```python
from build123d import *

# Parameters (mm, degrees)
EXTRUDE_DEPTH = 3.3
SKETCH001_R   = 1.5
POCKET_DEPTH  = 3.301
PAD_DEPTH     = 1


with BuildPart() as part:
    # Sketch → Extrude (new body)
    with BuildSketch(Plane.XY):
        with BuildLine():
            ThreePointArc((3.5, 21.5), (0, 25), (-3.5, 21.5))
            Line((-3.5, 21.5), (-3.5, 19.691369))
            ThreePointArc((-3.5, 19.691369), (0, -20), (3.5, 19.691369))
            Line((3.5, 19.691369), (3.5, 21.5))
        make_face()
    extrude(amount=EXTRUDE_DEPTH)

    # Sketch001 (on Face6 of Extrude) → Pocket (cut, through all)
    with BuildSketch(Plane.XY.offset(3.3)):
        with Locations((0, 21.5)):
            Circle(SKETCH001_R)
    extrude(amount=-POCKET_DEPTH, mode=Mode.SUBTRACT)

    # Sketch002 (on Face1 of CopyClone) → Pad (join)
    with BuildSketch(Plane.XY.offset(3.3)):
        with BuildLine():
            Line((-1.5, 13.5), (-1.5, -5))
            ThreePointArc((-1.5, -5), (0, -6.5), (1.5, -5))
            Line((1.5, 13.5), (1.5, -5))
            ThreePointArc((1.5, 13.5), (0, 14.581139), (-1.5, 13.5))
        make_face()
        with BuildLine():
            Line((-3.2, 9.765466), (-3.2, 6.765466))
            ThreePointArc((-3.2, 6.765466), (0, -10.943698), (3.2, 6.765466))
            Line((3.2, 9.765466), (3.2, 6.765466))
            ThreePointArc((-3.2, 9.765466), (0, -13.8), (3.2, 9.765466))
        make_face()
    extrude(amount=PAD_DEPTH)


solid = part.part
```
Build history of the part. All positions in model axes, mm. A direction names the side the tool comes from. Give positions to 0.01 mm unless a question says otherwise; leave off trailing zeros. Order: outer loops, then holes, each group sorted by start corner. A loop starts at its lowest first (then second) coordinate and runs counter-clockwise, first axis right, second up. Notation, with made-up numbers: M -39.75,55 L -12.75,55 A24 ccw -12.75,74 Z; hole C 70.5,76 d10. An arc over 180 degrees is marked long. Return JSON: item names as keys, results as strings.
Q1. 3-axis set-ups, long thin cutter, end or side, ignore diameter. For faces 4 (the face through (-0.83, -19.983, 1.627)), 5 (the face through (3.2, 8, 4)), 6 (the face through (-3.5, 21, 2)), 7 (the face through (-0.48, -13.79, 3.79)): which of +Z, -Z, +X, -X, +Y, -Y reach the whole face in a straight line?
Answer list:
{"face 4": "+Z, -Z", "face 5": "+Z, +Y", "face 6": "+Z, -Z, -X, +Y", "face 7": "+Z"}
Q2. Wall check: probe 1 along X at (y, z) = (-1.8, 3.75); probe 2 along Y at (x, z) = (0, 1.1); probe 3 along Z at (x, y) = (-6.5, 1). Give the ranges that are in metal, low to high. Write a range as from..to.
Answer list:
{"probe 1": "x = -12..-9.14, -1.5..1.5, 9.14..12", "probe 2": "y = -20..20, 23..25", "probe 3": "z = 0..3.3"}
Q3. Flat gauge pins, fed straight in: pin 1 (12 mm diameter, centred on x = 3.5, y = -13.5, fed in from -Z); pin 2 (0.5 mm diameter, centred on y = 20.5, z = 2, fed in from +X); pin 3 (0.5 mm diameter, centred on y = 8.5, z = 4, fed in from +X); pin 4 (0.5 mm diameter, centred on y = 6, z = 4, fed in from -X). Where does each tip first touch, or does it go through?
Answer list:
{"pin 1": "stops at z = 0", "pin 2": "stops at x = 3.5", "pin 3": "stops at x = 6.56", "pin 4": "stops at x = -9.33"}
Q4. Band-saw the part on D-D (x = -11). Give the cut face in (y, z).
Answer list:
{"outline": "M -16.7,0 L 16.7,0 L 16.7,3.3 L 3,3.3 L 3,4.3 L -6.6,4.3 L -6.6,3.3 L -16.7,3.3 Z"}
Q5. Band-saw the part on B-B (z = 0.8). Give the cut face in (x, y).
Answer list:
{"outline": "M -3.5,19.69 A20 ccw long 3.5,19.69 L 3.5,21.5 A3.5 ccw -3.5,21.5 Z; hole C 0,21.5 d3"}
Q6. Two-plate mould, pull along X, no slides. Class faces 1 (the face through (3.5, 21, 2)), 2 (the face through (0, 25, 2)), 3 (the face through (0, -6.5, 3.8)): pulls with the +X half, pulls with the -X half, needs draft (parallel to the pull), parting line crosses it, or undercut.
Answer list:
{"face 1": "pulls with the +X half", "face 2": "parting line crosses it", "face 3": "undercut"}
Q7. Band-saw the part on A-A (x = 0). Give the cut face in (y, z), then the cut area to 3 significant figures.
Answer list:
{"outline": "M -20,0 L 20,0 L 20,3.3 L 14.58,3.3 L 14.58,4.3 L -6.5,4.3 L -6.5,3.3 L -10.94,3.3 L -10.94,4.3 L -13.8,4.3 L -13.8,3.3 L -20,3.3 Z; M 23,0 L 25,0 L 25,3.3 L 23,3.3 Z", "area": "163 mm^2"}
Q8. Band-saw the part on C-C (y = 0). Give the cut face in (x, z), then the cut area to 3 significant figures.
Answer list:
{"outline": "M -20,0 L 20,0 L 20,3.3 L 11.86,3.3 L 11.86,4.3 L 8.96,4.3 L 8.96,3.3 L 1.5,3.3 L 1.5,4.3 L -1.5,4.3 L -1.5,3.3 L -8.96,3.3 L -8.96,4.3 L -11.86,4.3 L -11.86,3.3 L -20,3.3 Z", "area": "141 mm^2"}
